Verification items for the finished model (mm, model axes). A direction names the side the tool comes from. Give positions to 0.01 mm unless a question says otherwise; leave off trailing zeros. Write each loop counter-clockwise with the first axis right and the second up, starting at its lowest first coordinate (ties: lowest second). Pieces come first, ordered by that corner, then holes. Notation, with made-up numbers: M 2.5,-27 L 44.5,-27 A20 ccw 44.5,-12 Z; hole C -9.75,75.5 d5. An arc over 180 degrees is marked long. Write item = value, one per line.
from build123d import *

# Parameters (mm, degrees)
F0_W     = 76.2
F0_H     = 136.525
F1_DEPTH = 31.75
F2_W     = 38.1
F2_H     = 136.525
F3_DEPTH = 12.7
F5_R     = 9.525
F6_DEPTH = 12.7
F4_R     = 3.175
F7_DEPTH = 254


with BuildPart() as f1:
    # F0 (on Top) → F1 (new body)
    with BuildSketch(Plane.XY):
        Rectangle(F0_W, F0_H)
    extrude(amount=F1_DEPTH)

    # F2 (on face) → F3 (cut)
    with BuildSketch(Plane.XY.offset(31.75)):
        Rectangle(F2_W, F2_H)
    extrude(amount=-F3_DEPTH, mode=Mode.SUBTRACT)

    # F5 (on face) → F6 (cut)
    with BuildSketch(Plane(origin=(0, 0, 0), x_dir=(1, 0, 0), z_dir=(0, 0, -1))):
        Circle(F5_R)
    extrude(amount=-F6_DEPTH, mode=Mode.SUBTRACT)

    # F4 (on face) → F7 (cut)
    with BuildSketch(Plane.XY.offset(19.05)):
        Circle(F4_R)
    extrude(amount=-F7_DEPTH, mode=Mode.SUBTRACT)


solid = f1.part
1) Cross-section at B-B on y = 0. Record the boundary of the cut face in (x, z) (3 decimals).
From the geometry:
outline = M -38.1,0 L -9.525,0 L -9.525,12.7 L -3.175,12.7 L -3.175,19.05 L -19.05,19.05 L -19.05,31.75 L -38.1,31.75 Z; M 3.175,12.7 L 9.525,12.7 L 9.525,0 L 38.1,0 L 38.1,31.75 L 19.05,31.75 L 19.05,19.05 L 3.175,19.05 Z
2) Tool access check on faces 5 (the flat face through (-29, 1, 31.75)), 6 (the flat face through (-19.05, -1, 25)), 7 (the cylindrical face through (-7.559, 5.796, 6.261)). Record the directions out of +Z, -Z, +X, -X, +Y, -Y that give a thin tool (end or side, any length) a straight path to the whole face; none if there is none.
From the geometry:
face_5 = +Z, +X, -X, +Y, -Y
face_6 = +Z, +Y, -Y
face_7 = -Z
3) Cross-section at D-D on y = -17. Record the boundary of the cut face in (x, z).
From the geometry:
outline = M -38.1,0 L 38.1,0 L 38.1,31.75 L 19.05,31.75 L 19.05,19.05 L -19.05,19.05 L -19.05,31.75 L -38.1,31.75 Z
4) Cross-section at A-A on z = 29. Record the boundary of the cut face in (x, y).
From the geometry:
outline = M -38.1,-68.26 L -19.05,-68.26 L -19.05,68.26 L -38.1,68.26 Z; M 19.05,-68.26 L 38.1,-68.26 L 38.1,68.26 L 19.05,68.26 Z
5) Material ranges on probe 1 along X at (y, z) = (-47, 22.5); probe 2 along Y at (x, z) = (0, 17.25) (1 decimal); probe 3 along X at (y, z) = (0, 9) (3 decimals), recorded low to high. Write a range as from..to.
From the geometry:
probe_1 = -38.1..-19.05, 19.05..38.1
probe_2 = -68.3..-3.2, 3.2..68.3
probe_3 = -38.1..-9.525, 9.525..38.1
6) Depth check by flat-ended pin: P1, Ø1, axis at x = 3.5, y = -16, coming from the +Z side. Enter the tip coordinate at first touch or a pass-through.
From the geometry:
P1 = 19.05
7) Draft check along X on faces 1 (the flat face through (38.1, -1, 16)), 2 (the flat face through (19.05, -1, 25)), 3 (the cylindrical face through (-0.69, -3.1, 15.92)), 4 (the flat face through (28, 1, 31.75)). Enter one of: +X half, -X half, draft (parallel to the pull), parting line (faces both ways), or undercut.
From the geometry:
face_1 = +X half
face_2 = undercut
face_3 = undercut
face_4 = draft
